```python
from build123d import *

# Parameters (mm, degrees)
EXTRUDE_1_DEPTH                  = 35
SKETCH_2_W                       = 22
SKETCH_2_H                       = 35
EXTRUDE_2_DEPTH                  = 22.75
SKETCH_3_W                       = 11
SKETCH_3_H                       = 15
CUT_EXTRUDE_1_DEPTH              = 32
HOLE_WIZARD_12_5_12_5_1_D        = 12.5
HOLE_WIZARD_12_5_12_5_2_D        = 12.5
HOLE_WIZARD_3_5_3_5_1_D          = 3.5
HOLE_WIZARD_3_5_3_5_1_DEPTH      = 5
SKETCH_10_W                      = 9.5
SKETCH_10_H                      = 18.75
CUT_EXTRUDE_2_DEPTH              = 64.639610362
SKETCH_11_W                      = 22.75
SKETCH_11_H                      = 11
CUT_EXTRUDE_3_DEPTH              = 15
FILLET_2_R                       = 10
SKETCH_13_W                      = 4
SKETCH_13_H                      = 30
EXTRUDE_3_DEPTH                  = 31
SKETCH_16_W                      = 1.75
SKETCH_16_H                      = 4
HOLE_WIZARD_3_5_3_5_2_AT_2_COUNT = 2
HOLE_WIZARD_3_5_3_5_2_AT_2_PITCH = 24
HOLE_WIZARD_3_5_3_5_2_AT_3_COUNT = 2
HOLE_WIZARD_3_5_3_5_2_AT_3_PITCH = 33.941125497
HOLE_WIZARD_3_5_3_5_2_AT_4_COUNT = 2
HOLE_WIZARD_3_5_3_5_2_AT_4_PITCH = 24
SKETCH_17_R                      = 14
CUT_EXTRUDE_4_DEPTH              = 76.494728698
SKETCH_19_W                      = 4
SKETCH_19_H                      = 30
EXTRUDE_5_DEPTH                  = 34
SKETCH_20_R                      = 14
CUT_EXTRUDE_5_DEPTH              = 76.494728698
SKETCH_22_W                      = 1.75
SKETCH_22_H                      = 4
HOLE_WIZARD_3_5_3_5_3_AT_2_COUNT = 2
HOLE_WIZARD_3_5_3_5_3_AT_2_PITCH = 24
HOLE_WIZARD_3_5_3_5_3_AT_3_COUNT = 2
HOLE_WIZARD_3_5_3_5_3_AT_3_PITCH = 33.941125497
HOLE_WIZARD_3_5_3_5_3_AT_4_COUNT = 2
HOLE_WIZARD_3_5_3_5_3_AT_4_PITCH = 24
EXTRUDE_6_DEPTH                  = 4
EXTRUDE_7_DEPTH                  = 4
SKETCH_26_W                      = 10
SKETCH_26_H                      = 4
EXTRUDE_8_DEPTH                  = 35
HOLE_WIZARD_3_5_3_5_4_D          = 3.5
FILLET_7_R                       = 2
FILLET_9_R                       = 5
FILLET_10_R                      = 10
FILLET_12_R                      = 10
FILLET_13_R                      = 2
FILLET_14_R                      = 2
CUT_EXTRUDE_6_DEPTH              = 86.007352664


# Some blends are built 0.0001 mm under size
with BuildPart() as part:
    # Sketch 1 → Extrude 1 (new body)
    with BuildSketch(Plane(origin=(0, 35, 0), x_dir=(1, 0, 0), z_dir=(0, 1, 0))):
        with BuildLine():
            Line((35, 0), (13, 0))
            Line((13, 0), (13, -28))
            ThreePointArc((13, -28), (16.514718626, -36.485281374), (25, -40))
            ThreePointArc((25, -40), (32.16515139, -35.913807126), (35, -28.167840434))
            Line((35, -28.167840434), (35, 0))
        make_face()
    extrude(amount=-EXTRUDE_1_DEPTH)

    # Sketch 2 → Extrude 2 (add)
    with BuildSketch(Plane.ZY.offset(-13)):
        with Locations((11, 17.5)):
            Rectangle(SKETCH_2_W, SKETCH_2_H)
    extrude(amount=EXTRUDE_2_DEPTH)

    # Sketch 3 → Cut-Extrude 1 (cut)
    with BuildSketch(Plane.ZY.offset(9.75)):
        with Locations((5.5, 7.5)):
            Rectangle(SKETCH_3_W, SKETCH_3_H)
    extrude(amount=-CUT_EXTRUDE_1_DEPTH, mode=Mode.SUBTRACT)

    # Hole Wizard 12.5 _12.5_1 (through all)
    with Locations(Plane(origin=(0, 35, 0), x_dir=(1, 0, 0), z_dir=(0, 1, 0))):
        with Locations((24, -29)):
            Hole(HOLE_WIZARD_12_5_12_5_1_D / 2)

    # Hole Wizard 12.5 _12.5_2 (through all)
    with Locations(Plane(origin=(35, 0, 0), x_dir=(0, 0, -1), z_dir=(1, 0, 0))):
        with Locations((-11, 25)):
            Hole(HOLE_WIZARD_12_5_12_5_2_D / 2)

    # Hole Wizard 3.5 _3.5_1
    with Locations(Plane(origin=(0, 15, 0), x_dir=(-1, 0, 0), z_dir=(0, -1, 0))):
        with Locations((-17.25, -7), (6.75, -7), (-12.25, -7), (1.75, -7)):
            Hole(HOLE_WIZARD_3_5_3_5_1_D / 2, depth=HOLE_WIZARD_3_5_3_5_1_DEPTH)

    # Sketch 10 → Cut-Extrude 2 (cut, through all)
    with BuildSketch(Plane.XZ):
        with Locations((30.25, 9.375)):
            Rectangle(SKETCH_10_W, SKETCH_10_H)
    extrude(amount=-CUT_EXTRUDE_2_DEPTH, mode=Mode.SUBTRACT)

    # Sketch 11 → Cut-Extrude 3 (cut)
    with BuildSketch(Plane.XZ):
        with Locations((1.625, 16.5)):
            Rectangle(SKETCH_11_W, SKETCH_11_H)
    extrude(amount=-CUT_EXTRUDE_3_DEPTH, mode=Mode.SUBTRACT)

    # Fillet 2
    fillet_2_edges = [part.edges().sort_by_distance(p)[0] for p in [
        (25, 17.5, 40),
    ]]
    fillet(fillet_2_edges, radius=FILLET_2_R)

    # Sketch 19 → Extrude 5 (add)
    with BuildSketch(Plane.ZY.offset(9.75)):
        with Locations((2, 7.5)):
            Rectangle(SKETCH_19_W, SKETCH_19_H)
    extrude(amount=EXTRUDE_5_DEPTH)

    # Sketch 20 → Cut-Extrude 5 (cut, through all)
    with BuildSketch(Plane.XY.offset(4)):
        with Locations((-28.75, 7.5)):
            Circle(SKETCH_20_R)
    extrude(amount=-CUT_EXTRUDE_5_DEPTH, mode=Mode.SUBTRACT)

    # Sketch 22 → Hole Wizard 3.5 _3.5_3 (revolve, cut)
    with BuildSketch(Plane(origin=(-16.75, 19.5, 4), x_dir=(0, -1, 0), z_dir=(1, 0, 0))):
        with Locations((0.875, 2)):
            Rectangle(SKETCH_22_W, SKETCH_22_H)
    hole_wizard_3_5_3_5_3 = revolve(axis=Axis((-16.75, 19.5, 10.35), (0, 0, -1)), mode=Mode.SUBTRACT)

    # Hole Wizard 3.5 _3.5_3 at 2: Hole Wizard 3.5 _3.5_3 ×2
    with Locations(*[(0, -i * HOLE_WIZARD_3_5_3_5_3_AT_2_PITCH, 0) for i in range(1, HOLE_WIZARD_3_5_3_5_3_AT_2_COUNT)]):
        add(hole_wizard_3_5_3_5_3, mode=Mode.SUBTRACT)

    # Hole Wizard 3.5 _3.5_3 at 3: Hole Wizard 3.5 _3.5_3 ×2
    with Locations(*[Vector(-0.7071067811865475, -0.7071067811865476, 0) * (i * HOLE_WIZARD_3_5_3_5_3_AT_3_PITCH) for i in range(1, HOLE_WIZARD_3_5_3_5_3_AT_3_COUNT)]):
        add(hole_wizard_3_5_3_5_3, mode=Mode.SUBTRACT)

    # Hole Wizard 3.5 _3.5_3 at 4: Hole Wizard 3.5 _3.5_3 ×2
    with Locations(*[(-i * HOLE_WIZARD_3_5_3_5_3_AT_4_PITCH, 0, 0) for i in range(1, HOLE_WIZARD_3_5_3_5_3_AT_4_COUNT)]):
        add(hole_wizard_3_5_3_5_3, mode=Mode.SUBTRACT)

    # Sketch 24 → Extrude 6 (add)
    with BuildSketch(Plane.XY.offset(4)):
        Polygon((-9.75, 30.5), (-17.75, 22.5), (-9.75, 22.5), align=None)
    extrude(amount=-EXTRUDE_6_DEPTH)



with BuildPart() as body_2:
    # Sketch 13 → Extrude 3 (new body)
    with BuildSketch(Plane(origin=(25.5, 0, 0), x_dir=(0, 0, -1), z_dir=(1, 0, 0))):
        with Locations((-2, 7.5)):
            Rectangle(SKETCH_13_W, SKETCH_13_H)
    extrude(amount=EXTRUDE_3_DEPTH)

    # Sketch 16 → Hole Wizard 3.5 _3.5_2 (revolve, cut)
    with BuildSketch(Plane(origin=(29.5, -4.5, 4), x_dir=(0, -1, 0), z_dir=(1, 0, 0))):
        with Locations((0.875, 2)):
            Rectangle(SKETCH_16_W, SKETCH_16_H)
    hole_wizard_3_5_3_5_2 = revolve(axis=Axis((29.5, -4.5, 10.35), (0, 0, -1)), mode=Mode.SUBTRACT)

    # Hole Wizard 3.5 _3.5_2 at 2: Hole Wizard 3.5 _3.5_2 ×2
    with Locations(*[(0, i * HOLE_WIZARD_3_5_3_5_2_AT_2_PITCH, 0) for i in range(1, HOLE_WIZARD_3_5_3_5_2_AT_2_COUNT)]):
        add(hole_wizard_3_5_3_5_2, mode=Mode.SUBTRACT)

    # Hole Wizard 3.5 _3.5_2 at 3: Hole Wizard 3.5 _3.5_2 ×2
    with Locations(*[Vector(0.7071067811865475, 0.7071067811865476, 0) * (i * HOLE_WIZARD_3_5_3_5_2_AT_3_PITCH) for i in range(1, HOLE_WIZARD_3_5_3_5_2_AT_3_COUNT)]):
        add(hole_wizard_3_5_3_5_2, mode=Mode.SUBTRACT)

    # Hole Wizard 3.5 _3.5_2 at 4: Hole Wizard 3.5 _3.5_2 ×2
    with Locations(*[(i * HOLE_WIZARD_3_5_3_5_2_AT_4_PITCH, 0, 0) for i in range(1, HOLE_WIZARD_3_5_3_5_2_AT_4_COUNT)]):
        add(hole_wizard_3_5_3_5_2, mode=Mode.SUBTRACT)

    # Sketch 17 → Cut-Extrude 4 (cut, through all)
    with BuildSketch(Plane.XY.offset(4)):
        with Locations((41.5, 7.5)):
            Circle(SKETCH_17_R)
    extrude(amount=-CUT_EXTRUDE_4_DEPTH, mode=Mode.SUBTRACT)


with BuildPart() as part_1:
    add(part.part)

    add(body_2.part)  # Extrude 7 merges body 2
    # Sketch 25 → Extrude 7 (add)
    with BuildSketch(Plane.XY.offset(4)):
        Polygon((33.5, 22.5), (25.5, 30.5), (25.5, 22.5), align=None)
    extrude(amount=-EXTRUDE_7_DEPTH)

    # Sketch 26 → Extrude 8 (add)
    with BuildSketch(Plane.XY.offset(22)):
        with Locations((5.25, 17)):
            Rectangle(SKETCH_26_W, SKETCH_26_H)
    extrude(amount=EXTRUDE_8_DEPTH)

    # Hole Wizard 3.5 _3.5_4 (through all)
    with Locations(Plane(origin=(0, 15, 0), x_dir=(-1, 0, 0), z_dir=(0, -1, 0))):
        with Locations((-5.25, -52), (-5.25, -42), (-5.25, -32)):
            Hole(HOLE_WIZARD_3_5_3_5_4_D / 2)

    # Fillet 7
    fillet_7_edges = [part_1.edges().sort_by_distance(p)[0] for p in [
        (0.25, 17, 22),
        (10.25, 17, 22),
    ]]
    fillet(fillet_7_edges, radius=FILLET_7_R)

    # Fillet 9
    fillet_9_edges = [part_1.edges().sort_by_distance(p)[0] for p in [
        (0.25, 17, 57),
        (10.25, 17, 57),
    ]]
    fillet(fillet_9_edges, radius=FILLET_9_R - 0.0001)  # a hair under: the kernel refuses the full size

    # Fillet 10
    # the kernel refuses this fillet: 10 mm, written as the material it takes off along each edge
    with BuildSketch(Plane(origin=(35, -32.046488893, 18.75), x_dir=(-0.03816406367220006, 0, 0.999271486756239), z_dir=(0, 1, 0))) as fillet_10_piece_1:
        with BuildLine():
            CenterArc((10.360556073, -9.693195649), FILLET_10_R, 75.770650452, 103.082689776)
            Line((0.362558605, -9.493079124), (-0.637241142, -9.473067472))
            ThreePointArc((-0.637241142, -9.473067472), (-0.817992184, -4.784703626), (-0.999271487, -0.038164064))
            Line((-0.999271487, -0.038164064), (-0.038164064, 0.999271487))
            ThreePointArc((-0.038164064, 0.999271487), (9.372815349, 1.358694549), (13.064399506, 0.969319565))
            Line((13.064399506, 0.969319565), (12.818595557, 0))
        make_face()
    extrude(amount=99.092977786, mode=Mode.SUBTRACT)

    # Fillet 12
    fillet_12_edges = [part_1.edges().sort_by_distance(p)[0] for p in [
        (1.625, 35, 22),
    ]]
    fillet(fillet_12_edges, radius=FILLET_12_R)

    # Fillet 13
    fillet_13_edges = [part_1.edges().sort_by_distance(p)[0] for p in [
        (-9.75, 30.5, 2),
        (-9.75, -7.5, 2),
        (-43.75, 22.5, 2),
        (-43.75, -7.5, 2),
        (-17.75, 22.5, 2),
    ]]
    fillet(fillet_13_edges, radius=FILLET_13_R)

    # Fillet 14
    fillet_14_edges = [part_1.edges().sort_by_distance(p)[0] for p in [
        (56.5, 22.5, 2),
        (25.5, 30.5, 2),
        (33.5, 22.5, 2),
        (25.5, -7.5, 2),
        (56.5, -7.5, 2),
    ]]
    fillet(fillet_14_edges, radius=FILLET_14_R)

    # Sketch 32 → Cut-Extrude 6 (cut, through all)
    with BuildSketch(Plane.XY.offset(4)):
        with BuildLine():
            Line((-9.75, 2.270340952), (-9.75, 15))
            ThreePointArc((-9.75, 15), (-10.952290213, 8.635170476), (-9.75, 2.270340952))
        make_face()
    extrude(amount=-CUT_EXTRUDE_6_DEPTH, mode=Mode.SUBTRACT)


solid = part_1.part
```
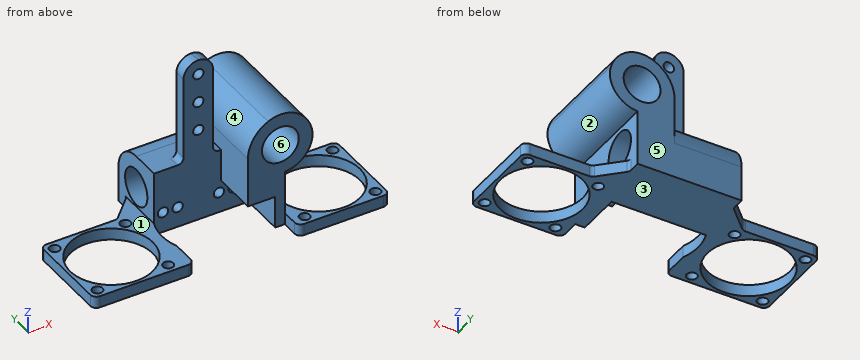
Verification items for the finished model (mm, model axes). Face numbers are marked on the shaded views. A direction names the side the tool comes from. Round coordinates to 2 decimals unless told otherwise and drop trailing zeros. Order: outer loops, then holes, each group sorted by start corner. A loop starts at its lowest first (then second) coordinate and runs counter-clockwise, first axis right, second up. Notation, with made-up numbers: (26.25, 21.5) - (43.25, 21.5) arc R19 cw to (43.25, 27.5) - close; hole circle Ø8 at (48.5, -1). An arc over 180 degrees is marked (long way). Use CSV: the item, a comma, the result in double quotes. Start each with the question number.
1) Section check B-B, the plane x = -28.75. Record the cut outline in (y, z), plus the area to 3 significant figures.
2) Section check D-D, the plane z = 26.5. Record the cut outline in (x, y).
3) Access from +Z, -Z, +X, -X, +Y, -Y to the whole of each face (thin tool, end or side, straight path). Record for the marked faces 1 and 2.
4) Thickness scan on L1, parallel to Z at x = 5.25, y = 16; L2, parallel to Y at x = -28.75, z = 1.25; L3, parallel to X at y = 17, z = 32. Record the ranges inside material, lowest first.
5) Section check A-A, the plane z = 42. Record the cut outline in (x, y), plus the area to 3 significant figures.
6) Section check C-C, the plane y = 12. State how many separate pieces and enclosed holes the cut face has, plus the area to 3 significant figures.
7) Go/stop test with flat-tipped pins: P1, Ø12, axis at y = 16.5, z = 22.5, coming from the +X side; P2, Ø1.2, axis at x = 45, z = 2, coming from the +Y side; P3, Ø4.5, axis at x = 15.5, y = 9.5, coming from the -Z side. Record where each tip stops, or that it passes through.
8) Mould release check, pull along Z, two halves, no side actions. Record for the marked faces 3, 4, 5 and 6: +Z half, -Z half, draft (parallel to the pull), parting line (faces both ways), or undercut.
Answers:
1,outline,"(-7.5, 0) - (-6.5, 0) - (-6.5, 4) - (-7.5, 4) - close; (21.5, 0) - (22.5, 0) - (22.5, 4) - (21.5, 4) - close"
1,area,"8.00 mm²"
2,outline,"(0.25, 15) - (10.25, 15) - (10.25, 19) - (0.25, 19) - close; (13, 0) - (18.27, 0) - (18.27, 35) - (13, 35) - close; (29.73, 0) - (34.67, 0) - (34.67, 35) - (29.73, 35) - close"
3,face 1,"+Z, -X, +Y, -Y"
3,face 2,"+X, +Y, -Y"
4,L1,"z = 0 to 30.25, 33.75 to 40.25, 43.75 to 50.25, 53.75 to 57"
4,L2,"y = -7.5 to -6.5, 21.5 to 22.5"
4,L3,"x = 0.25 to 3.5, 7 to 10.25, 13.69 to 18.52, 29.48 to 34.37"
5,outline,"(0.25, 15) - (3.5, 15) - (3.5, 19) - (0.25, 19) - close; (7, 15) - (10.25, 15) - (10.25, 19) - (7, 19) - close"
5,area,"26.0 mm²"
6,separate pieces,"4"
6,enclosed holes,"1"
6,area,"439 mm²"
7,P1,"stops at x = 34.92"
7,P2,"stops at y = 22.5"
7,P3,"stops at z = 11"
8,face 3,"-Z half"
8,face 4,"+Z half"
8,face 5,"draft"
8,face 6,"undercut"
